Design review of the part built by this model. Coordinates are the model's own, in mm. Face numbers are marked on the shaded views. A direction names the side the tool comes from. Coordinates: 2 decimals unless noted, no trailing zeros. Loops run counter-clockwise (first coordinate to the right, second up) from the corner with the lowest first, then second, coordinate; pieces in that order, holes last. Notation, with made-up numbers: M 34.5,44.25 L 47.5,44.25 A15 cw 47.5,60.25 Z; hole C 12.25,76 d1. An arc over 180 degrees is marked long. Answer as a JSON object with one key per item and string values. Group by question number.
1. Consider section B-B (z = 17.5). State the section outline as (x, y) points, then the cut area to 3 significant figures.
2. Draft analysis for pull direction X (two halves, no side actions). For the marked faces 4, 5 and 6, state which applies: +X half, -X half, draft (parallel to the pull), parting line (faces both ways), or undercut.
3. Consider section A-A (x = -3). State the section outline as (y, z) points.
4. Consider section C-C (x = -25). State the section outline as (y, z) points, then the cut area to 3 significant figures.
5. Consider section D-D (y = 2.7). Count the separate pieces of the cut face and the enclosed holes in it, then the cut area to 3 significant figures.
6. To check wall thickness, follow probe 1 along Z at (x, y) = (-9.75, 4.5); probe 2 along Z at (x, y) = (-13, 1); probe 3 along Z at (x, y) = (-4.5, 4.75). State the ranges of each line that lie inside material, in increasing order.
7. Insertion check: pin 1 (3.5 mm diameter, centred on x = -3.5, y = 4.5, fed in from +Z); pin 2 (3 mm diameter, centred on x = -9.5, y = 4, fed in from +Z) (3 decimals); pin 3 (3 mm diameter, centred on y = 2.5, z = 17.5, fed in from -X); pin 4 (2 mm diameter, centred on x = -3, y = 4.5, fed in from -Z). Each pin has a flat end and moves straight along its axis. Give the tip position at first contact, or say it passes through.
8. Machinability: for the marked faces 1, 2 and 3, which of the approach directions +Z, -Z, +X, -X, +Y, -Y give a long, thin tool a straight path to every point of the face, cutting with its end or side? Answer none if there is none.
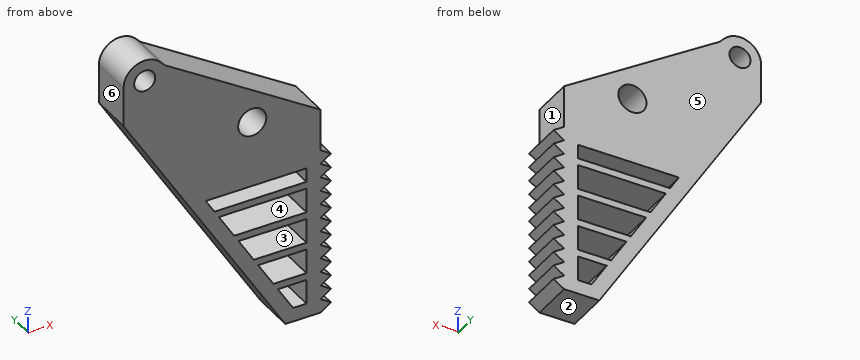
from build123d import *

# Parameters (mm, degrees)
EXTRUDE_1_DEPTH        = 6
CUT_EXTRUDE_1_DEPTH    = 58.619441164
SKETCH_3_W             = 4.685619361
SKETCH_3_H             = 1
SKETCH_3_W_2           = 7.482916658
SKETCH_3_W_3           = 10.280213956
SKETCH_3_W_4           = 13.077511253
EXTRUDE_1_2_DEPTH      = 6
EXTRUDE_2_DEPTH        = 6
PATTERN_LINEAR_1_COUNT = 12
PATTERN_LINEAR_1_PITCH = 2
FILLET_3_R             = 3
SKETCH_5_R             = 1.5
SKETCH_5_R_2           = 2
CUT_EXTRUDE_2_DEPTH    = 54.92122199


with BuildPart() as part:
    # 草图1 → Extrude 1 (new body)
    with BuildSketch(Plane(origin=(0, 0, 0), x_dir=(1, 0, 0), z_dir=(0, 1, 0))):
        Polygon((0, 0), (-5, 0), (-28, -37), (-28, -50), (-22.078758581, -44), (0, -30), align=None)
    extrude(amount=EXTRUDE_1_DEPTH)

    # 草图2 → 切除-拉伸1 (cut, through all)
    with BuildSketch(Plane(origin=(0, 6, 0), x_dir=(1, 0, 0), z_dir=(0, 1, 0))):
        Polygon((-3.888322064, -2), (-2, -2), (-2, -22), (-16.320754496, -22), align=None)
    extrude(amount=-CUT_EXTRUDE_1_DEPTH, mode=Mode.SUBTRACT)

    # 草图3 → Extrude 1 2 (add)
    with BuildSketch(Plane(origin=(0, 6, 0), x_dir=(1, 0, 0), z_dir=(0, 1, 0))):
        with Locations((-4.342809681, -6)):
            Rectangle(SKETCH_3_W, SKETCH_3_H)
        with Locations((-5.741458329, -10.5)):
            Rectangle(SKETCH_3_W_2, SKETCH_3_H)
        with Locations((-7.140106978, -15)):
            Rectangle(SKETCH_3_W_3, SKETCH_3_H)
        with Locations((-8.538755627, -19.5)):
            Rectangle(SKETCH_3_W_4, SKETCH_3_H)
    extrude(amount=-EXTRUDE_1_2_DEPTH)

    # 草图4 → 凸台-拉伸2 (add)
    with BuildSketch(Plane(origin=(0, 6, 0), x_dir=(1, 0, 0), z_dir=(0, 1, 0))):
        Polygon((0, 0), (1.5, -1), (0, -2), align=None)
    extrude_2 = extrude(amount=-EXTRUDE_2_DEPTH)

    # 阵列(线性)1: 凸台-拉伸2 ×12
    with Locations(*[(0, 0, i * PATTERN_LINEAR_1_PITCH) for i in range(1, PATTERN_LINEAR_1_COUNT)]):
        add(extrude_2)

    # 圆角3
    fillet_3_edges = [part.edges().sort_by_distance(p)[0] for p in [
        (-28, 3, 50),
    ]]
    fillet(fillet_3_edges, radius=FILLET_3_R)

    # 草图5 → 切除-拉伸2 (cut, through all)
    with BuildSketch(Plane(origin=(0, 6, 0), x_dir=(1, 0, 0), z_dir=(0, 1, 0))):
        with Locations(Location((-25, -42.689147299, 0), (0, 0, 270))):
            Circle(SKETCH_5_R)
        with Locations(Location((-9.704707061, -31.417323404, 0), (0, 0, 270))):
            Circle(SKETCH_5_R_2)
    extrude(amount=-CUT_EXTRUDE_2_DEPTH, mode=Mode.SUBTRACT)


solid = part.part
Findings below:
{
 "1": {"outline": "M -15.88,0 L -13.52,0 L -13.52,6 L -15.88,6 Z; M -2,0 L 0.75,0 L 0.75,6 L -2,6 Z", "area": "30.6 mm^2"},
 "2": {"face 4": "undercut", "face 5": "draft", "face 6": "-X half"},
 "3": {"outline": "M 0,0 L 6,0 L 6,2 L 0,2 Z; M 0,5.5 L 6,5.5 L 6,6.5 L 0,6.5 Z; M 0,10 L 6,10 L 6,11 L 0,11 Z; M 0,14.5 L 6,14.5 L 6,15.5 L 0,15.5 Z; M 0,19 L 6,19 L 6,20 L 0,20 Z; M 0,22 L 6,22 L 6,31.9 L 0,31.9 Z"},
 "4": {"outline": "M 0,32.17 L 6,32.17 L 6,41.19 L 0,41.19 Z; M 0,44.19 L 6,44.19 L 6,45.69 L 0,45.69 Z", "area": "63.1 mm^2"},
 "5": {"separate pieces": "1", "enclosed holes": "7", "area": "529 mm^2"},
 "6": {"probe 1": "z = 7.64 to 11.43, 14.5 to 15.5, 19 to 20, 22 to 29.42, 33.42 to 36.18", "probe 2": "z = 12.87 to 16.66, 19 to 20, 22 to 38.24", "probe 3": "z = 0 to 2.98, 5.5 to 6.5, 10 to 11, 14.5 to 15.5, 19 to 20, 22 to 32.85"},
 "7": {"pin 1": "stops at z = 33.33", "pin 2": "stops at z = 36.975", "pin 3": "stops at x = -16.81", "pin 4": "stops at z = 0"},
 "8": {"face 1": "+Z, +X, +Y, -Y", "face 2": "-Z, +X, -X, +Y, -Y", "face 3": "+Y, -Y"}
}
